Check sheet for the modelled part. Datum: model origin and axes. Units: mm. Face numbers are marked on the shaded views. A direction names the side the tool comes from. Round coordinates to 2 decimals unless told otherwise and drop trailing zeros. Order: outer loops, then holes, each group sorted by start corner. A loop starts at its lowest first (then second) coordinate and runs counter-clockwise, first axis right, second up. Notation, with made-up numbers: M 40,75.25 L 67,75.25 A22 cw 67,94.25 Z; hole C 77,45.5 d2. An arc over 180 degrees is marked long. One line per item, written item: value. Start each with the question number.
(1) Access from +Z, -Z, +X, -X, +Y, -Y to the whole of each face (thin tool, end or side, straight path). Record for the marked faces 5, 6, 7 and 8.
(2) Cross-section at A-A, the plane x = 0. Count the separate pieces of the cut face and the enclosed holes in it, and give its area (3 significant figures).
(3) Depth check by flat-ended pin: pin 1 Ø12 at (x, z) = (4, -6) entering from -Y; pin 2 Ø6.5 at (y, z) = (11, 0.5) entering from -X; pin 3 Ø6.5 at (x, z) = (-0.5, 0) entering from +Y; pin 4 Ø3 at (x, y) = (-1.5, 5) entering from -Z. Enter the tip coordinate at first touch or a pass-through.
(4) Release check for a two-part mould opening along Y. For the marked faces 1, 2, 3 and 4 record: released by +Y, released by -Y, zero draft, split by the parting line, or undercut.
(5) Cross-section at D-D, the plane z = -24. Enter the section's corners in (x, y) (3 decimals).
(6) Cross-section at C-C, the plane x = 20. Enter the section's corners in (y, z), and give its area (3 significant figures).
(7) Thickness scan on L1, parallel to X at y = 14.7, z = 0; L2, parallel to X at y = 10.75, z = 0; L3, parallel to Y at x = 25, z = 0. Record the ranges inside material, lowest first.
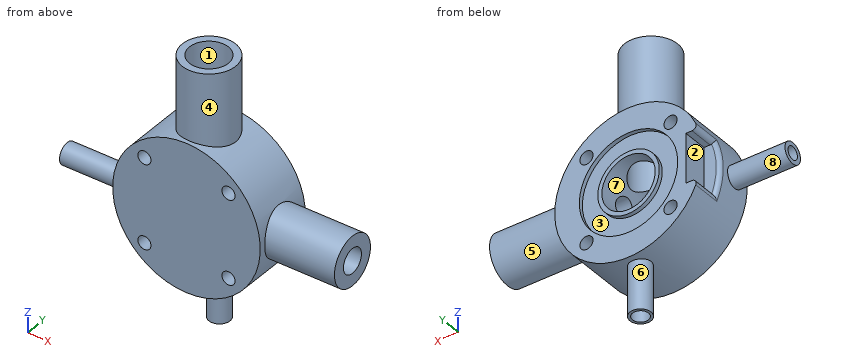
from build123d import *

# Parameters (mm, degrees)
SKETCH1_R         = 18
BODY_DEPTH        = 15
SKETCH2_R         = 12
SKETCH2_R_2       = 7.5
GASKET_DEPTH      = 1
SKETCH6_R         = 6
CE_PORT_DEPTH     = 35
SKETCH8_W         = 8
SKETCH8_H         = 12
SPE_DEPTH         = 6
SPE_FILLET_R      = 1
SKETCH9_R         = 6.5
RE_PORT_DEPTH     = 35
SKETCH10_R        = 4.75
RE_HOLE_DEPTH     = 35
SKETCH7_R         = 3
CE_HOLE_DEPTH     = 35
SKETCH11_R        = 1.6
BOLTS_DEPTH       = 35
SKETCH13_R        = 2.575
OUTLET_DEPTH      = 30
SKETCH4_R         = 6.5
CELL_VOL_DEPTH    = 13
OUTLET_H_R        = 1.963591437
OUTLET_HOLE_DEPTH = 30
SKETCH15_R        = 2.575
INLET_DEPTH       = 18
SKETCH16_R        = 1.575
INLET_HOLE_DEPTH  = 32


with BuildPart() as part:
    # Sketch1 → Body (new body)
    with BuildSketch(Plane(origin=(0, 0, 0), x_dir=(1, 0, 0), z_dir=(0, 1, 0))):
        with Locations(Location((0, 0, 0), (0, 0, 270))):
            Circle(SKETCH1_R)
    extrude(amount=BODY_DEPTH)

    # Sketch2 → Gasket (cut)
    with BuildSketch(Plane(origin=(0, 15, 0), x_dir=(1, 0, 0), z_dir=(0, 1, 0))):
        with Locations(Location((0, 0, 0), (0, 0, 270))):
            Circle(SKETCH2_R)
        with Locations(Location((0, 0, 0), (0, 0, 270))):
            Circle(SKETCH2_R_2, mode=Mode.SUBTRACT)
    extrude(amount=-GASKET_DEPTH, mode=Mode.SUBTRACT)

    # Sketch6 → CE_port (add)
    with BuildSketch(Plane(origin=(0, 0, 0), x_dir=(0, 0, -1), z_dir=(1, 0, 0))):
        with Locations(Location((0, 7.5, 0), (0, 0, 180))):
            Circle(SKETCH6_R)
    extrude(amount=CE_PORT_DEPTH)

    # Sketch8 → SPE (cut)
    with BuildSketch(Plane(origin=(0, 15, 0), x_dir=(1, 0, 0), z_dir=(0, 1, 0))):
        with Locations((-18, 0)):
            Rectangle(SKETCH8_W, SKETCH8_H)
    extrude(amount=-SPE_DEPTH, mode=Mode.SUBTRACT)

    # SPE_Fillet
    # the kernel refuses this fillet: 1 mm, written as the material it takes off along each edge
    with BuildSketch(Plane(origin=(0, 9, 0), x_dir=(-0.8875777915854841, 0, 0.4606578598962953), z_dir=(0.4606578598962953, 0, 0.8875777915854841))) as spe_fillet_piece_1_section:
        with BuildLine():
            CenterArc((18 - SPE_FILLET_R, SPE_FILLET_R), SPE_FILLET_R, 270, 90)
            Line((18 - SPE_FILLET_R, 0), (18, 0))
            Line((18, 0), (18, SPE_FILLET_R))
        make_face()
    spe_fillet_piece_1 = revolve(axis=Axis((0, 9, 0), (0, -1, 0)), revolution_arc=54.859132299, mode=Mode.PRIVATE)
    spe_fillet_piece_1 = split(spe_fillet_piece_1, bisect_by=Plane(origin=(-17.717440744, 8.717440744, 6), z_dir=(0, 0, -1)), keep=Keep.TOP, mode=Mode.PRIVATE)
    spe_fillet_piece_1 = split(spe_fillet_piece_1, bisect_by=Plane(origin=(-17.717440744, 8.717440744, -6), z_dir=(0, 0, 1)), keep=Keep.TOP, mode=Mode.PRIVATE)
    add(spe_fillet_piece_1, mode=Mode.SUBTRACT)
    with BuildSketch(Plane(origin=(-16.970562748, 18.803742657, -6), x_dir=(0.3728821950274604, 0, -0.9278786928427136), z_dir=(0, -1, 0))) as spe_fillet_piece_2:
        with BuildLine():
            CenterArc((1.479233256, 0.999106486), SPE_FILLET_R, 158.106520097, 114.315739171)
            Line((0.551354563, 1.371988681), (0, 0))
            ThreePointArc((0, 0), (0.760748531, -0.01608325), (1.521497063, 0))
        make_face()
    extrude(amount=9.803742657, mode=Mode.SUBTRACT)
    with BuildSketch(Plane(origin=(-16.970562748, 18.803742657, 6), x_dir=(0.37288219502746, 0, 0.9278786928427138), z_dir=(0, -1, 0))) as spe_fillet_piece_3:
        with BuildLine():
            CenterArc((1.479233256, -0.999106486), SPE_FILLET_R, 87.577740732, 114.315739171)
            Line((0.551354563, -1.371988681), (0, 0))
            ThreePointArc((0, 0), (0.760748531, 0.01608325), (1.521497063, 0))
        make_face()
    extrude(amount=9.803742657, mode=Mode.SUBTRACT)
    with BuildSketch(Plane(origin=(-16.970562748, 18.803742657, 6), x_dir=(0.37288219502746, 0, 0.9278786928427138), z_dir=(0, -1, 0))) as spe_fillet_piece_4a_section:
        with BuildLine():
            CenterArc((1.479233256, -0.999106486), SPE_FILLET_R, 87.577740732, 114.315739171)
            Line((0.551354563, -1.371988681), (0, 0))
            ThreePointArc((0, 0), (0.760748531, 0.01608325), (1.521497063, 0))
        make_face()
    spe_fillet_piece_4a = extrude(amount=13.607485314, mode=Mode.PRIVATE)
    spe_fillet_piece_4a = split(spe_fillet_piece_4a, bisect_by=Plane(origin=(-16.491409341, 9, 6.340012755), z_dir=(0, -1, 0)), keep=Keep.TOP, mode=Mode.PRIVATE)
    with BuildSketch(Plane(origin=(0, 9, 0), x_dir=(-0.8875777915854841, 0, 0.4606578598962953), z_dir=(0.4606578598962953, 0, 0.8875777915854841))) as spe_fillet_piece_4b_section:
        with BuildLine():
            CenterArc((18 - SPE_FILLET_R, SPE_FILLET_R), SPE_FILLET_R, 270, 90)
            Line((18 - SPE_FILLET_R, 0), (18, 0))
            Line((18, 0), (18, SPE_FILLET_R))
        make_face()
    spe_fillet_piece_4b = revolve(axis=Axis((0, 9, 0), (0, -1, 0)), revolution_arc=54.859132299, mode=Mode.PRIVATE)
    spe_fillet_piece_4b = split(spe_fillet_piece_4b, bisect_by=Plane(origin=(-16.286739391, 8.767935426, 6), z_dir=(0, 0, 1)), keep=Keep.TOP, mode=Mode.PRIVATE)
    spe_fillet_piece_4 = spe_fillet_piece_4a & spe_fillet_piece_4b
    add(spe_fillet_piece_4, mode=Mode.SUBTRACT)
    with BuildSketch(Plane(origin=(0, 9, 0), x_dir=(-0.8875777915854841, 0, 0.4606578598962953), z_dir=(0.4606578598962953, 0, 0.8875777915854841))) as spe_fillet_piece_5a_section:
        with BuildLine():
            CenterArc((18 - SPE_FILLET_R, SPE_FILLET_R), SPE_FILLET_R, 270, 90)
            Line((18 - SPE_FILLET_R, 0), (18, 0))
            Line((18, 0), (18, SPE_FILLET_R))
        make_face()
    spe_fillet_piece_5a = revolve(axis=Axis((0, 9, 0), (0, -1, 0)), revolution_arc=54.859132299, mode=Mode.PRIVATE)
    spe_fillet_piece_5a = split(spe_fillet_piece_5a, bisect_by=Plane(origin=(-16.286739653, 8.767935416, -6), z_dir=(0, 0, -1)), keep=Keep.TOP, mode=Mode.PRIVATE)
    with BuildSketch(Plane(origin=(-16.970562748, 18.803742657, -6), x_dir=(0.3728821950274604, 0, -0.9278786928427136), z_dir=(0, -1, 0))) as spe_fillet_piece_5b_section:
        with BuildLine():
            CenterArc((1.479233256, 0.999106486), SPE_FILLET_R, 158.106520097, 114.315739171)
            Line((0.551354563, 1.371988681), (0, 0))
            ThreePointArc((0, 0), (0.760748531, -0.01608325), (1.521497063, 0))
        make_face()
    spe_fillet_piece_5b = extrude(amount=13.607485314, mode=Mode.PRIVATE)
    spe_fillet_piece_5b = split(spe_fillet_piece_5b, bisect_by=Plane(origin=(-16.491409341, 9, -6.340012755), z_dir=(0, -1, 0)), keep=Keep.TOP, mode=Mode.PRIVATE)
    spe_fillet_piece_5 = spe_fillet_piece_5a & spe_fillet_piece_5b
    add(spe_fillet_piece_5, mode=Mode.SUBTRACT)

    # Sketch9 → RE_port (add)
    with BuildSketch(Plane.XY):
        with Locations(Location((0, 7.5, 0), (0, 0, 180))):
            Circle(SKETCH9_R)
    extrude(amount=RE_PORT_DEPTH)

    # Sketch10 → RE_hole (cut)
    with BuildSketch(Plane.XY.offset(35)):
        with Locations((0, 7.5)):
            Circle(SKETCH10_R)
    extrude(amount=-RE_HOLE_DEPTH, mode=Mode.SUBTRACT)

    # Sketch7 → CE_hole (cut)
    with BuildSketch(Plane(origin=(35, 0, 0), x_dir=(0, 0, -1), z_dir=(1, 0, 0))):
        with Locations((0, 7.5)):
            Circle(SKETCH7_R)
    extrude(amount=-CE_HOLE_DEPTH, mode=Mode.SUBTRACT)

    # Sketch11 → Bolts (cut)
    with BuildSketch(Plane(origin=(0, 15, 0), x_dir=(1, 0, 0), z_dir=(0, 1, 0))):
        with Locations(Location((-10.253048327, 10.253048327, 0), (0, 0, 270))):
            Circle(SKETCH11_R)
        with Locations(Location((10.253048327, 10.253048327, 0), (0, 0, 270))):
            Circle(SKETCH11_R)
        with Locations(Location((10.253048327, -10.253048327, 0), (0, 0, 270))):
            Circle(SKETCH11_R)
        with Locations(Location((-10.253048327, -10.253048327, 0), (0, 0, 270))):
            Circle(SKETCH11_R)
    extrude(amount=-BOLTS_DEPTH, mode=Mode.SUBTRACT)

    # Sketch13 → Outlet (add)
    with BuildSketch(Plane.XY):
        with Locations((0, 11)):
            Circle(SKETCH13_R)
    extrude(amount=-OUTLET_DEPTH)

    # Sketch4 → Cell_vol (cut)
    with BuildSketch(Plane(origin=(0, 15, 0), x_dir=(1, 0, 0), z_dir=(0, 1, 0))):
        with Locations(Location((0, 0, 0), (0, 0, 270))):
            Circle(SKETCH4_R)
    extrude(amount=-CELL_VOL_DEPTH, mode=Mode.SUBTRACT)

    # Outlet_h → Outlet_hole (cut)
    with BuildSketch(Plane(origin=(0, 0, -30), x_dir=(-1, 0, 0), z_dir=(0, 0, -1))):
        with Locations((0, 11)):
            Circle(OUTLET_H_R)
    extrude(amount=-OUTLET_HOLE_DEPTH, mode=Mode.SUBTRACT)

    # Sketch15 → Inlet (add)
    with BuildSketch(Plane.ZY.offset(14)):
        with Locations(Location((0, 4, 0), (0, 0, 180))):
            Circle(SKETCH15_R)
    extrude(amount=INLET_DEPTH)

    # Sketch16 → Inlet_hole (cut)
    with BuildSketch(Plane.ZY.offset(32)):
        with Locations((0, 4)):
            Circle(SKETCH16_R)
    extrude(amount=-INLET_HOLE_DEPTH, mode=Mode.SUBTRACT)


solid = part.part
Values found:
1. face 5: +X
1. face 6: -Z
1. face 7: +Y
1. face 8: -X
2. separate pieces: 3
2. enclosed holes: 0
2. area: 282 mm^2
3. pin 1: y = 0
3. pin 2: x = -18
3. pin 3: y = 2
3. pin 4: z = -18
4. face 1: undercut
4. face 2: zero draft
4. face 3: released by +Y
4. face 4: split by the parting line
5. outline: C 0,11 d5.15; hole C 0,11 d3.927
6. outline: C 7.5,0 d12; hole C 7.5,0 d6
6. area: 84.8 mm^2
7. L1: -14 to -12, -7.5 to -6.5, 6.5 to 7.5, 12 to 18
7. L2: -14 to -6.5, 6.5 to 35
7. L3: 1.5 to 4.5, 10.5 to 13.5
